from build123d import *

# Parameters (mm, degrees)
ESQUISSE1_R        = 1.5
BOSS_EXTRU_1_DEPTH = 5


with BuildPart() as part:
    # Esquisse1 → Boss.-Extru.1 (new body)
    with BuildSketch(Plane.XY):
        with BuildLine():
            ThreePointArc((-30.851851852, 40.60989088), (-43.125037525, 27.225560389), (-49.930555556, 10.389399497))
            ThreePointArc((-49.930555556, 10.389399497), (-43.743567635, 11.431158196), (-37.930555556, 9.070444049))
            ThreePointArc((-37.930555556, 9.070444049), (-32.666503706, 21.304918109), (-23.592592593, 31.054622438))
            ThreePointArc((-23.592592593, 31.054622438), (-22.444588001, 39.461886289), (-30.851851852, 40.60989088))
        make_face()
        with Locations((-27.222222222, 35.832256659)):
            Circle(ESQUISSE1_R, mode=Mode.SUBTRACT)
        Polygon((-41.654998366, 20.666666667), (-37.175966284, 18.444444444), (-32.731521839, 27.402508609), (-37.210553922, 29.624730831), align=None, mode=Mode.SUBTRACT)
    extrude(amount=BOSS_EXTRU_1_DEPTH)


solid = part.part
Here's how the part is built. I have some questions about the finished solid (model axes, mm). A direction names the side the tool comes from. Round coordinates to 2 decimals unless told otherwise and drop trailing zeros. Order: outer loops, then holes, each group sorted by start corner. A loop starts at its lowest first (then second) coordinate and runs counter-clockwise, first axis right, second up. Notation, with made-up numbers: M 80.5,75 L 115.5,75 A26 cw 115.5,109 Z; hole C -38,20.25 d7. An arc over 180 degrees is marked long. Return JSON: item names as keys, results as strings. Group by question number.
1. If we section it at C-C on z = 4.4: List the corners of the cut face in (x, y) for me (1 decimal).
2. If we mould it in two halves opening along X, with no side actions, what happens to faces 1 (the face through (-27.55, 34.37, 2.46)), 2 (the face through (-22.4, 39.4, 2.5)), 3 (the face through (-33, 26, 0)), 4 (the face through (-43.83, 11.44, 2.46))? For each: pulls with the +X half, pulls with the -X half, needs draft (parallel to the pull), parting line crosses it, or undercut.
3. I'm going to push flat-ended pins straight in: pin 1 Ø1.5 at (x, z) = (-46, 1.5) entering from +Y; pin 2 Ø1.5 at (y, z) = (34, 0.5) entering from +X. Where does each tip first touch, or does it pass through?
4. On a 3-axis mill with a long thin cutter (end or side, diameter ignored), from which of +Z, -Z, +X, -X, +Y, -Y can I reach the whole of each face in a straight line? I mean faces 5 (the face through (-42.99, 27.44, 2.46)), 6 (the face through (-34.94, 28.5, 2.46)). Say none if no direction works.
5. Please list where these lines run through material, in increasing order: probe 1 along X at (y, z) = (21, 2.45); probe 2 along X at (y, z) = (26, 0.65); probe 3 along Y at (x, z) = (-28.25, 3.35).
6. If we section it at A-A on x = -35: List the corners of the cut face in (y, z) for me, then the cut area to 3 significant figures.
7. If we section it at D-D on x = -44: List the corners of the cut face in (y, z) for me.
8. If we section it at B-B on y = 28.5: List the corners of the cut face in (x, z) for me.
Reply:
{
 "1": {"outline": "M -49.9,10.4 A11.5 cw -37.9,9.1 A39 cw -23.6,31.1 A6 ccw -30.9,40.6 A51 ccw Z; hole M -41.7,20.7 L -37.2,18.4 L -32.7,27.4 L -37.2,29.6 Z; hole C -27.2,35.8 d3"},
 "2": {"face 1": "undercut", "face 2": "parting line crosses it", "face 3": "needs draft", "face 4": "undercut"},
 "3": {"pin 1": "y = 23.53", "pin 2": "x = -21.32"},
 "4": {"face 5": "+Z, -Z, -X, +Y", "face 6": "+Z, -Z"},
 "5": {"probe 1": "-46.48 to -41.49, -35.91 to -32.86", "probe 2": "-43.87 to -39.01, -33.43 to -29.07", "probe 3": "26.89 to 34.74, 36.92 to 41.74"},
 "6": {"outline": "M 17.2,0 L 22.83,0 L 22.83,5 L 17.2,5 Z; M 28.53,0 L 37.09,0 L 37.09,5 L 28.53,5 Z", "area": "71.0 mm^2"},
 "7": {"outline": "M 11.46,0 L 25.79,0 L 25.79,5 L 11.46,5 Z"},
 "8": {"outline": "M -42.29,0 L -37.77,0 L -37.77,5 L -42.29,5 Z; M -34.94,0 L -26.62,0 L -26.62,5 L -34.94,5 Z"}
}
